from build123d import *

# Parameters (mm, degrees)
SKETCH_W           = 18.5
SKETCH_H           = 18.5
SKETCH_R           = 8.15
PAD_DEPTH          = 4
SKETCH001_W        = 18.5
SKETCH001_H        = 18.5
PAD001_DEPTH       = 3
SKETCH002_R        = 9.25
SKETCH003_R        = 5.4
SKETCH005_R        = 5.4
PAD002_DEPTH       = 2
CHAMFER_SIZE       = 1.5
CHAMFER001_SIZE    = 1.5
POCKET_DEPTH       = 120.882639
POLARPATTERN_COUNT = 4
SKETCH007_R        = 4.4
SKETCH008_R        = 5.4


with BuildPart() as part:
    # Sketch → Pad (new body)
    with BuildSketch(Plane.XY):
        Rectangle(SKETCH_W, SKETCH_H)
        Circle(SKETCH_R, mode=Mode.SUBTRACT)
    extrude(amount=PAD_DEPTH)

    # Sketch001 (on Face7 of Pad) → Pad001 (join)
    with BuildSketch(Plane.XY.offset(4)):
        Rectangle(SKETCH001_W, SKETCH001_H)
    extrude(amount=PAD001_DEPTH)

    # Sketch002 (on Face10 of Pad001) → AdditiveLoft section 0
    with BuildSketch(Plane.XY.offset(7)):
        Circle(SKETCH002_R)
    # Sketch003 (on Face10 of Pad001) → AdditiveLoft section 1
    with BuildSketch(Plane.XY.offset(42)):
        Circle(SKETCH003_R)
    loft()

    # Sketch005 (on Face17 of AdditiveLoft) → Pad002 (join)
    with BuildSketch(Plane.XY.offset(42)):
        Circle(SKETCH005_R)
    extrude(amount=PAD002_DEPTH)

    # Chamfer
    chamfer_edges = [part.edges().sort_by_distance(p)[0] for p in [
        (-9.25, -9.25, 5.5),
        (-9.25, -9.25, 2),
        (9.25, -9.25, 5.5),
        (9.25, -9.25, 2),
        (9.25, 9.25, 2),
        (9.25, 9.25, 5.5),
        (-9.25, 9.25, 5.5),
        (-9.25, 9.25, 2),
    ]]
    chamfer(chamfer_edges, length=CHAMFER_SIZE)

    # Chamfer001
    chamfer001_edges = [part.edges().sort_by_distance(p)[0] for p in [
        (8.5, -8.5, 7),
        (-8.5, -8.5, 7),
        (-8.5, 8.5, 7),
        (8.5, 8.5, 7),
    ]]
    chamfer(chamfer001_edges, length=CHAMFER001_SIZE)

    # Sketch006 (on Face19 of Chamfer001) → Pocket (cut, through all)
    with BuildSketch(Plane.YZ.offset(9.25)):
        Polygon((0, 42), (-2.7, 7), (2.7, 7), align=None)
    pocket = extrude(amount=-POCKET_DEPTH, mode=Mode.SUBTRACT)

    # PolarPattern: Pocket ×4 about axis
    polarpattern_axis = Axis((0, 0, 0), (0, 0, 1))
    for i in range(1, POLARPATTERN_COUNT):
        add(pocket.rotate(polarpattern_axis, i * 360 / POLARPATTERN_COUNT), mode=Mode.SUBTRACT)

    # Sketch007 (on Face47 of PolarPattern) → AdditiveLoft001 section 0
    with BuildSketch(Plane.XY.offset(44)):
        Circle(SKETCH007_R)
    # Sketch008 → AdditiveLoft001 section 1
    with BuildSketch(Plane.XY.offset(46)):
        Circle(SKETCH008_R)
    loft()


solid = part.part
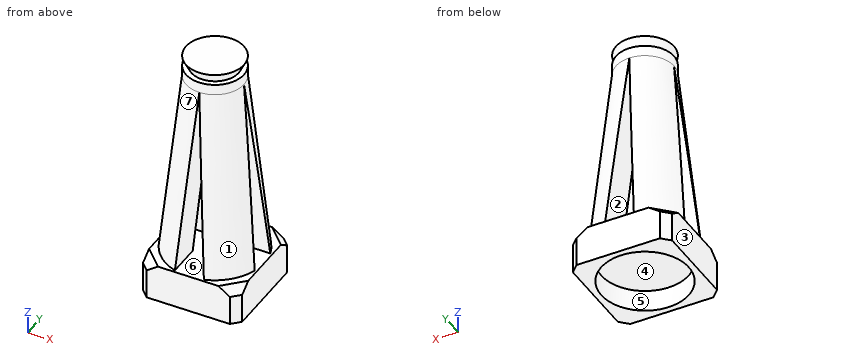
Can you work these out from the model? Positions are in its coordinate system, mm. Face numbers are marked on the shaded views. A direction names the side the tool comes from. Round coordinates to 2 decimals unless told otherwise and drop trailing zeros. Write each loop counter-clockwise with the first axis right and the second up, starting at its lowest first coordinate (ties: lowest second). Pieces come first, ordered by that corner, then holes. Notation, with made-up numbers: (69.5, 76) - (105.5, 76) arc R16 ccw to (105.5, 107) - close; hole circle Ø10 at (-23, 7.5). An arc over 180 degrees is marked (long way). Write each question's results on one line, items separated by ' | '. Start each with the question number.
1) We'd pull the mould along Z, two halves only. Please class the marked faces 1, 2, 3 and 4: released by +Z, released by -Z, zero draft, split by the parting line, or undercut.
2) Suppose I cut it at B-B (z = 41.5). List the corners of the cut face in (x, y) for me (3 decimals), and give its area (3 significant figures).
3) Which directions (+Z, -Z, +X, -X, +Y, -Y) give clear straight access to the entire face, cutting with the end or side of a thin tool? Please do the marked faces 5, 6 and 7.
4) For pin 1 Ø10 at (y, z) = (1.5, 22.5) entering from +X; pin 2 Ø6 at (y, z) = (-5.5, 19.5) entering from +X; pin 3 Ø1.5 at (x, y) = (7.5, 7) entering from +Z, each with a flat end and sliding along its axis, tell me the tip position at first contact or that it passes through.
5) Suppose I cut it at A-A (z = 15.5). List the corners of the cut face in (x, y) for me (3 decimals).
6) Please list where these lines run through material, in increasing order: line 1 (Y direction, x = 0, z = 1.65); line 2 (X direction, y = -3.25, z = 21.5); line 3 (Z direction, x = -7.25, y = 6.25).
Here are the results:
1) face 1: released by +Z | face 2: undercut | face 3: zero draft | face 4: released by -Z
2) outline: (-5.455, -0.039) arc R5.455 ccw to (-0.039, -5.455) - (-0.039, -0.039) - close; (-5.455, 0.039) - (-0.039, 0.039) - (-0.039, 5.455) arc R5.455 ccw to start; (0.039, -5.455) arc R5.455 ccw to (5.455, -0.039) - (0.039, -0.039) - close; (0.039, 0.039) - (5.455, 0.039) arc R5.455 ccw to (0.039, 5.455) - close | area: 91.8 mm2
3) face 5: -Z | face 6: none | face 7: +Z, -X, -Y
4) pin 1: stops at x = 7.87 | pin 2: stops at x = 7.53 | pin 3: stops at z = 7
5) outline: (-8.06, -2.044) arc R8.315 ccw to (-2.044, -8.06) - (-2.044, -2.044) - close; (-8.06, 2.044) - (-2.044, 2.044) - (-2.044, 8.06) arc R8.315 ccw to start; (2.044, -8.06) arc R8.315 ccw to (8.06, -2.044) - (2.044, -2.044) - close; (2.044, 2.044) - (8.06, 2.044) arc R8.315 ccw to (2.044, 8.06) - close
6) line 1: y = -9.25 to -8.15, 8.15 to 9.25 | line 2: x = -6.93 to -1.58, 1.58 to 6.93 | line 3: z = 0 to 7
